The drawing under review shows one solid part. Ordinate dimensions are in mm from its lowest x, y, z. A direction names the side the tool comes from. Coordinates: 2 decimals unless noted, no trailing zeros. Loops run counter-clockwise (first coordinate to the right, second up) from the corner with the lowest first, then second, coordinate; pieces in that order, holes last. Notation, with made-up numbers: (72.25, 65) - (85.25, 65) arc R17 ccw to (85.25, 92) - close; hole circle Ø3 at (48, 55). An arc over 180 degrees is marked (long way). Answer as a JSON object with one key per item and string values. Group by question number.
Item 1: To check wall thickness, follow line 1 (Z direction, x = 153, y = 7) (1 decimal); line 2 (Z direction, x = 72.5, y = 9) (1 decimal); line 3 (X direction, y = 7.75, z = 35) (1 decimal). State the ranges of each line that lie inside material, in increasing order.
Item 2: Mouldability with a two-part tool opening along X and no side actions: class the marked faces 5, 6 and 7 as released by +X, released by -X, zero draft, split by the parting line, or undercut.
Item 3: We need section B-B (x = 130). Give the boundary of the cut face in (y, z), then the cut area to 3 significant figures.
Item 4: Clearance check with flat-ended pins moving along their axes: pin 1 (12 mm diameter, centred on y = 9, z = 90.5, fed in from -X); pin 2 (12 mm diameter, centred on x = 138, y = 6, fed in from -Z); pin 3 (8 mm diameter, centred on y = 5, z = 138, fed in from +X); pin 4 (11 mm diameter, centred on y = 13, z = 142, fed in from -X) (1 decimal). State where each tip first meets the part, or that it passes through.
Item 5: We need section C-C (y = 16.75). Give the boundary of the cut face in (x, z).
Item 6: Tool access review of the marked faces 1, 2, 3 and 4: name each direction out of +Z, -Z, +X, -X, +Y, -Y from which nothing blocks a thin tool from reaching the whole face with its end or side.
Item 7: We need section A-A (z = 131). Give the boundary of the cut face in (x, y).
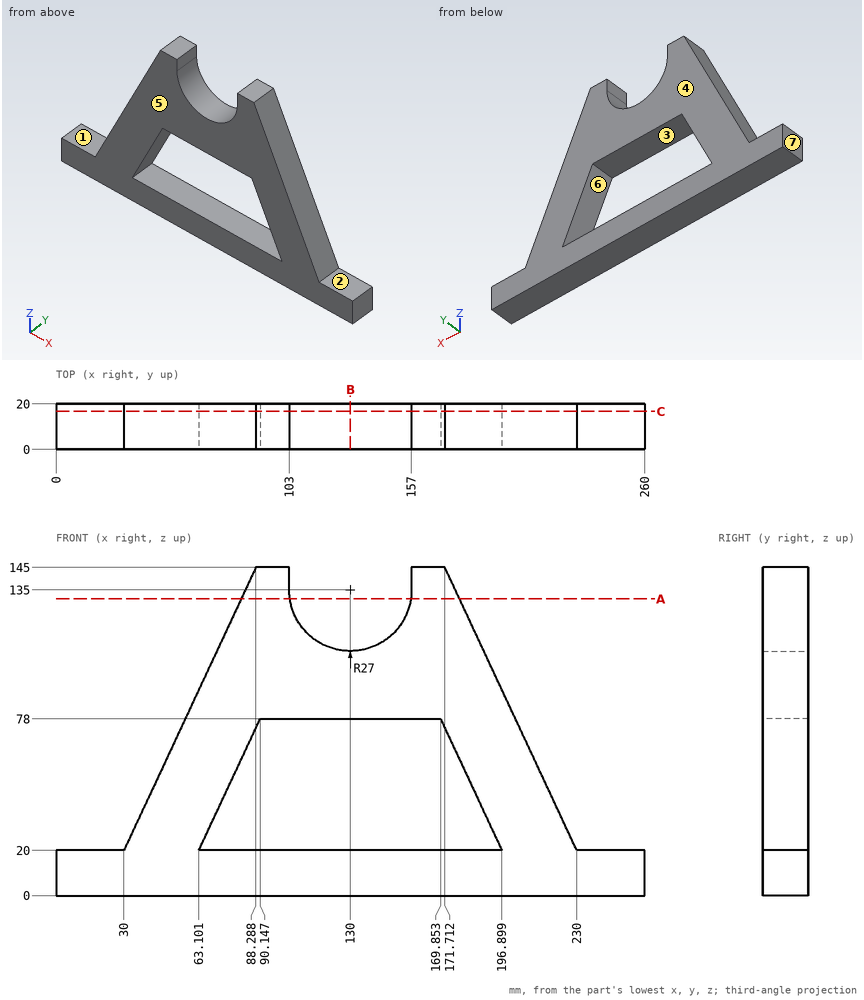
Check sheet entries:
{
 "1": {"line 1": "z = 0 to 20, 78 to 120.9", "line 2": "z = 0 to 20, 40.2 to 111.1", "line 3": "x = 37 to 70.1, 189.9 to 223"},
 "2": {"face 5": "zero draft", "face 6": "undercut", "face 7": "released by -X"},
 "3": {"outline": "(0, 0) - (20, 0) - (20, 20) - (0, 20) - close; (0, 78) - (20, 78) - (20, 108) - (0, 108) - close", "area": "1,000 mm2"},
 "4": {"pin 1": "stops at x = 60.08", "pin 2": "stops at z = 0", "pin 3": "stops at x = 176.84", "pin 4": "stops at x = 84.3"},
 "5": {"outline": "(0, 0) - (260, 0) - (260, 20) - (230, 20) - (171.71, 145) - (157, 145) - (157, 135) arc R27 cw to (103, 135) - (103, 145) - (88.29, 145) - (30, 20) - (0, 20) - close; hole (63.1, 20) - (196.9, 20) - (169.85, 78) - (90.15, 78) - close"},
 "6": {"face 1": "+Z, -X, +Y, -Y", "face 2": "+Z, +X, +Y, -Y", "face 3": "+Y, -Y", "face 4": "+Z, -Z, +X, -X, +Y"},
 "7": {"outline": "(81.76, 0) - (103.3, 0) - (103.3, 20) - (81.76, 20) - close; (156.7, 0) - (178.24, 0) - (178.24, 20) - (156.7, 20) - close"}
}
